Autodesk Inventor part; units mm, degrees
ref_plane "YZ Plane" through (0, 0, 0) normal (1, 0, 0) x (0, 1, 0)
ref_plane "XZ Plane" through (0, 0, 0) normal (0, 1, 0) x (-1, 0, 0)
ref_plane "XY Plane" through (0, 0, 0) normal (0, 0, 1) x (1, 0, 0)
sketch "スケッチ1" plane through (0, 0, 0) normal (0, 0, 1) x (1, 0, 0)
  spline S0 degree 4 poles (-46.7287, -62.3958) (-46.4075, -62.5897) (-45.9582, -62.8581) (-45.3809, -63.1982) (-44.6755, -63.6062) (-44.164, -63.8983) (-43.6533, -64.1863) (-43.1431, -64.4703) (-42.6335, -64.7504) (-42.1242, -65.0266) (-41.6152, -65.299) (-41.1064, -65.5676) (-40.5978, -65.8326) (-40.0892, -66.0938) (-39.5807, -66.3514) (-39.072, -66.6054) (-38.5633, -66.8559) (-38.0543, -67.1029) (-37.5452, -67.3463) (-37.0357, -67.5863) (-36.526, -67.8228) (-36.0159, -68.0558) (-35.5054, -68.2855) (-34.9944, -68.5118) (-34.483, -68.7346) (-33.9711, -68.9542) (-33.4587, -69.1703) (-32.9457, -69.3831) (-32.4322, -69.5925) (-31.9181, -69.7986) (-31.4034, -70.0014) (-30.8881, -70.2009) (-30.3721, -70.397) (-29.8555, -70.5898) (-29.3383, -70.7793) (-28.8203, -70.9655) (-28.3017, -71.1484) (-27.7825, -71.3279) (-27.2625, -71.5041) (-26.7419, -71.6771) (-26.2205, -71.8467) (-25.6985, -72.0129) (-25.1758, -72.1759) (-24.6524, -72.3355) (-24.1283, -72.4918) (-23.6035, -72.6447) (-23.078, -72.7943) (-22.5519, -72.9406) (-22.0251, -73.0835) (-21.4976, -73.2231) (-20.9695, -73.3593) (-20.4407, -73.4921) (-19.9113, -73.6216) (-19.3812, -73.7477) (-18.8505, -73.8704) (-18.3193, -73.9897) (-17.7874, -74.1057) (-17.2549, -74.2182) (-16.7219, -74.3274) (-16.1883, -74.4332) (-15.6541, -74.5355) (-15.1195, -74.6344) (-14.5843, -74.7299) (-14.0486, -74.822) (-13.5124, -74.9107) (-12.9757, -74.9959) (-12.4386, -75.0776) (-11.901, -75.156) (-11.363, -75.2309) (-10.8247, -75.3023) (-10.2859, -75.3703) (-9.7467, -75.4348) (-9.2072, -75.4958) (-8.6674, -75.5534) (-8.1272, -75.6075) (-7.5868, -75.6581) (-7.046, -75.7053) (-6.5051, -75.749) (-5.9638, -75.7892) (-5.4224, -75.8259) (-4.8807, -75.8591) (-4.3389, -75.8888) (-3.7969, -75.915) (-3.2547, -75.9378) (-2.7125, -75.957) (-2.1701, -75.9728) (-1.6276, -75.985) (-1.0851, -75.9938) (-0.5426, -75.999) (0, -76.0008) (0.5426, -75.999) (1.0851, -75.9938) (1.6276, -75.985) (2.1701, -75.9728) (2.7124, -75.957) (3.2547, -75.9378) (3.7969, -75.915) (4.3388, -75.8888) (4.8807, -75.8591) (5.4223, -75.8259) (5.9638, -75.7892) (6.505, -75.749) (7.046, -75.7053) (7.5867, -75.6582) (8.1271, -75.6075) (8.6672, -75.5534) (9.207, -75.4958) (9.7465, -75.4348) (10.2856, -75.3703) (10.8243, -75.3023) (11.3626, -75.2309) (11.9005, -75.156) (12.4379, -75.0777) (12.9749, -74.9959) (13.5114, -74.9108) (14.0474, -74.8221) (14.5829, -74.7301) (15.1179, -74.6346) (15.6524, -74.5357) (16.1862, -74.4334) (16.7195, -74.3277) (17.2522, -74.2186) (17.7843, -74.1061) (18.3158, -73.9902) (18.8466, -73.871) (19.3768, -73.7483) (19.9062, -73.6223) (20.435, -73.493) (20.9632, -73.3602) (21.4905, -73.2242) (22.0172, -73.0848) (22.5431, -72.9421) (23.0683, -72.796) (23.5927, -72.6466) (24.1163, -72.4939) (24.6392, -72.3379) (25.1612, -72.1786) (25.6825, -72.0161) (26.2029, -71.8502) (26.7225, -71.681) (27.2413, -71.5086) (27.7593, -71.3329) (28.2764, -71.154) (28.7926, -70.9718) (29.308, -70.7863) (29.8225, -70.5976) (30.3362, -70.4057) (30.849, -70.2105) (31.3609, -70.0121) (31.8719, -69.8105) (32.3821, -69.6057) (32.8914, -69.3976) (33.3998, -69.1863) (33.9073, -68.9719) (34.414, -68.7542) (34.9198, -68.5333) (35.4247, -68.3093) (35.9288, -68.082) (36.432, -67.8516) (36.9344, -67.6179) (37.4359, -67.381) (37.9366, -67.141) (38.4364, -66.8977) (38.9355, -66.6513) (39.4337, -66.4016) (39.9312, -66.1488) (40.4279, -65.8927) (40.9238, -65.6334) (41.419, -65.3709) (41.9135, -65.1051) (42.4073, -64.8361) (42.9004, -64.5639) (43.3928, -64.2884) (43.8846, -64.0096) (44.3758, -63.7275) (44.8664, -63.4421) (45.3565, -63.1534) (46.0301, -62.7516) (46.5798, -62.4176) (47.0065, -62.1545) (47.3109, -61.9649) knots 0 0 0 0 0 0.014459 0.020221 0.025968 0.031703 0.037425 0.043135 0.048834 0.054523 0.060202 0.065871 0.071532 0.077184 0.082829 0.088465 0.094095 0.099718 0.105334 0.110945 0.11655 0.122149 0.127744 0.133333 0.138918 0.144499 0.150076 0.155648 0.161217 0.166783 0.172345 0.177904 0.183461 0.189014 0.194565 0.200113 0.205659 0.211203 0.216745 0.222285 0.227822 0.233359 0.238893 0.244426 0.249957 0.255487 0.261016 0.266543 0.272069 0.277594 0.283118 0.288641 0.294163 0.299685 0.305205 0.310725 0.316243 0.321762 0.327279 0.332796 0.338313 0.343828 0.349344 0.354859 0.360373 0.365887 0.371401 0.376914 0.382427 0.38794 0.393452 0.398964 0.404476 0.409988 0.415499 0.421011 0.426522 0.432033 0.437544 0.443054 0.448565 0.454075 0.459586 0.465096 0.470606 0.476117 0.481627 0.487137 0.492647 0.498157 0.503667 0.509177 0.514688 0.520198 0.525708 0.531218 0.536729 0.542239 0.54775 0.553261 0.558771 0.564282 0.569793 0.575304 0.580816 0.586327 0.591839 0.597351 0.602863 0.608375 0.613888 0.6194 0.624913 0.630427 0.63594 0.641454 0.646969 0.652483 0.657998 0.663514 0.66903 0.674546 0.680063 0.68558 0.691098 0.696617 0.702136 0.707656 0.713176 0.718697 0.724219 0.729741 0.735265 0.740789 0.746314 0.75184 0.757367 0.762895 0.768424 0.773955 0.779486 0.785019 0.790553 0.796089 0.801626 0.807165 0.812705 0.818247 0.82379 0.829336 0.834883 0.840433 0.845984 0.851538 0.857094 0.862653 0.868214 0.873778 0.879345 0.884914 0.890487 0.896063 0.901642 0.907224 0.912811 0.918401 0.923995 0.929593 0.935196 0.940803 0.946414 0.952031 0.957653 0.96328 0.968913 0.974552 0.980196 0.985847 1 1 1 1 1
  arc A0 (-43.3371, -57.4602) -> (-46.7287, -62.3958) centre (-45.1853, -59.8233) ccw
  arc A1 (-43.3371, -57.4602) -> (-12.9977, -50.3865) centre (-31.0158, -41.7063) ccw
  arc A2 (12.8817, -50.3865) -> (43.8031, -57.1163) centre (30.9439, -41.7983) ccw
  arc A3 (47.3109, -61.9649) -> (43.8031, -57.1163) centre (45.732, -59.414) ccw
  arc A4 (-42.105, -55.8848) -> (-14.7995, -49.5185) centre (-31.0158, -41.7063) ccw
  arc A5 (-42.105, -55.8848) -> (-47.7601, -64.1093) centre (-45.1853, -59.8233) ccw
  arc A6 (48.3661, -63.6639) -> (42.5172, -55.5845) centre (45.732, -59.414) ccw
  arc A7 (14.6879, -49.5277) -> (42.5172, -55.5845) centre (30.9439, -41.7983) ccw
  line L0 (-12.9977, -50.3865) -> (-14.7995, -49.5185)
  line L1 (12.8817, -50.3865) -> (14.6879, -49.5277)
  spline S1 degree 5 poles (-47.7621, -64.1081) (-39.0585, -69.3622) (-29.7722, -73.6606) (-19.8779, -76.6074) (0.4344, -79.4943) (20.7174, -76.4) (30.5408, -73.3687) (39.7688, -69.0175) (48.3682, -63.6626) knots 0 0 0 0 0 0 0.500897 0.500897 0.500897 1 1 1 1 1 1
  point P0 (0, 0)
  point P1 (0, 0)
  dimension "d0" = 2
extrude "押し出し1" add sketch "スケッチ1" along normal blind 5
properties part number "脚ゴム2" material "ゴム、シリコーン"
Design review of the part built by this model. Coordinates are the model's own, in mm. A direction names the side the tool comes from. Coordinates: 2 decimals unless noted, no trailing zeros. Order: outer loops, then holes, each group sorted by start corner. A loop starts at its lowest first (then second) coordinate and runs counter-clockwise, first axis right, second up. Notation, with made-up numbers: (79, -5) - (86, -5) arc R8 cw to (86, 8) - close; hole circle Ø6 at (35, -31). An arc over 180 degrees is marked (long way). Put each result on its own line as item: value.
1) Take a section at A-A, the plane y = -53. Give the boundary of the cut face in (x, z), and give its area (3 significant figures).
Response values:
outline: (-17, 0) - (-14.51, 0) - (-14.51, 5) - (-17, 5) - close; (14.38, 0) - (16.85, 0) - (16.85, 5) - (14.38, 5) - close
area: 24.8 mm²
2) The part is to be moulded in two halves that separate along X. For faces 1 (the face through (48.12, -57.6, 2.46)), 2 (the face through (0, -77, 0)), say which applies: released by +X, released by -X, zero draft, split by the parting line, or undercut.
Response values:
face 1: undercut
face 2: zero draft
3) Insertion check: P1, Ø8, axis at x = -4.5, y = -72, coming from the +Z side; P2, Ø2, axis at x = 37.5, z = 3, coming from the -Y side; P3, Ø3, axis at y = -57.5, z = 1.5, coming from the -X side; P4, Ø3, axis at y = -66, z = 1.5, coming from the +X side. Each pin has a flat end and moves straight along its axis. Give the tip position at first contact, or say it passes through.
Response values:
P1: stops at z = 5
P2: stops at y = -70.02
P3: stops at x = -50.12
P4: stops at x = 47
4) Tool access review of faces 3 (the face through (-13.886, -49.959, 2.465)), 4 (the face through (26.941, -61.394, 2.465)), 5 (the face through (0, -77, 5)): name each direction out of +Z, -Z, +X, -X, +Y, -Y from which nothing blocks a thin tool from reaching the whole face with its end or side.
Response values:
face 3: +Z, -Z, +Y
face 4: +Z, -Z
face 5: +Z, +X, -X, +Y, -Y
5) Wall thickness on L1, parallel to X at y = -58.25, z = 0.45; L2, parallel to X at y = -55.5, z = 3.3; L3, parallel to X at y = -57.5, z = 1.35: over which ranges is each line inside the solid? List them lowest first. Write a range as from..to.
Response values:
L1: x = -49.93..-47.74, -42.25..-38.11, -23.92..-19.78, 19.57..23.64, 38.25..42.32, 48.5..50.59
L2: x = -47.7..-42.67, -19.45..-16.53, 16.37..19.27, 42.62..48.84
L3: x = -49.61..-47.08, -43.29..-39.65, -22.38..-18.75, 18.56..22.14, 39.74..43.33, 48.04..50.35
